from build123d import *

# Parameters (mm, degrees)
SKETCH1_R           = 23
SKETCH1_R_2         = 18
BOSS_EXTRUDE1_DEPTH = 11
SKETCH1_13_R        = 23
SKETCH1_13_R_2      = 18
SKETCH1_13_R_3      = 3
SKETCH1_13_R_4      = 5.25
BOSS_EXTRUDE2_DEPTH = 3
BOSS_EXTRUDE4_START = 3
SKETCH1_16_R        = 23
SKETCH1_16_R_2      = 18
SKETCH1_16_R_3      = 3
SKETCH1_16_R_4      = 5.25
SKETCH1_16_R_5      = 1.5
BOSS_EXTRUDE4_DEPTH = 3
SKETCH1_17_R        = 23
SKETCH1_17_R_2      = 18
BOSS_EXTRUDE5_DEPTH = 60
SKETCH2_R           = 1.5
CUT_EXTRUDE1_DEPTH  = 5
BOSS_EXTRUDE6_START = 6
SKETCH1_20_R        = 3
SKETCH1_20_R_2      = 1.5
BOSS_EXTRUDE6_DEPTH = 3
SKETCH1_21_R        = 23
SKETCH1_21_R_2      = 18
CUT_EXTRUDE4_DEPTH  = 23
SKETCH2_2_R         = 1.5
CUT_EXTRUDE5_DEPTH  = 9


with BuildPart() as part:
    # Sketch1 → Boss-Extrude1 (new body)
    with BuildSketch(Plane(origin=(0, 0, 0), x_dir=(0, 0, -1), z_dir=(1, 0, 0))):
        Circle(SKETCH1_R)
        Circle(SKETCH1_R_2, mode=Mode.SUBTRACT)
    extrude(amount=-BOSS_EXTRUDE1_DEPTH)

    # Sketch1_13 → Boss-Extrude2 (add)
    with BuildSketch(Plane(origin=(0, 0, 0), x_dir=(0, 0, -1), z_dir=(1, 0, 0))):
        Circle(SKETCH1_13_R)
        Circle(SKETCH1_13_R_2, mode=Mode.SUBTRACT)
        Circle(SKETCH1_13_R_2)
        with Locations((-8.5, 0)):
            Circle(SKETCH1_13_R_3, mode=Mode.SUBTRACT)
        with Locations((8.5, 0)):
            Circle(SKETCH1_13_R_3, mode=Mode.SUBTRACT)
        Circle(SKETCH1_13_R_4, mode=Mode.SUBTRACT)
        with Locations((0, -8.5)):
            Circle(SKETCH1_13_R_3, mode=Mode.SUBTRACT)
        with Locations((0, 8.5)):
            Circle(SKETCH1_13_R_3, mode=Mode.SUBTRACT)
    extrude(amount=BOSS_EXTRUDE2_DEPTH)

    # Sketch1_16 → Boss-Extrude4 (add)
    with BuildSketch(Plane(origin=(0, 0, 0), x_dir=(0, 0, -1), z_dir=(1, 0, 0)).offset(BOSS_EXTRUDE4_START)):
        Circle(SKETCH1_16_R)
        Circle(SKETCH1_16_R_2, mode=Mode.SUBTRACT)
        Circle(SKETCH1_16_R_2)
        with Locations((-8.5, 0)):
            Circle(SKETCH1_16_R_3, mode=Mode.SUBTRACT)
        with Locations((8.5, 0)):
            Circle(SKETCH1_16_R_3, mode=Mode.SUBTRACT)
        Circle(SKETCH1_16_R_4, mode=Mode.SUBTRACT)
        with Locations((0, -8.5)):
            Circle(SKETCH1_16_R_3, mode=Mode.SUBTRACT)
        with Locations((0, 8.5)):
            Circle(SKETCH1_16_R_3, mode=Mode.SUBTRACT)
        with Locations((0, 8.5)):
            Circle(SKETCH1_16_R_3)
        with Locations((0, 8.5)):
            Circle(SKETCH1_16_R_5, mode=Mode.SUBTRACT)
        with Locations((-8.5, 0)):
            Circle(SKETCH1_16_R_3)
        with Locations((-8.5, 0)):
            Circle(SKETCH1_16_R_5, mode=Mode.SUBTRACT)
        with Locations((0, -8.5)):
            Circle(SKETCH1_16_R_3)
        with Locations((0, -8.5)):
            Circle(SKETCH1_16_R_5, mode=Mode.SUBTRACT)
        with Locations((8.5, 0)):
            Circle(SKETCH1_16_R_3)
        with Locations((8.5, 0)):
            Circle(SKETCH1_16_R_5, mode=Mode.SUBTRACT)
    extrude(amount=BOSS_EXTRUDE4_DEPTH)

    # Sketch1_17 → Boss-Extrude5 (add)
    with BuildSketch(Plane(origin=(0, 0, 0), x_dir=(0, 0, -1), z_dir=(1, 0, 0))):
        Circle(SKETCH1_17_R)
        Circle(SKETCH1_17_R_2, mode=Mode.SUBTRACT)
    extrude(amount=BOSS_EXTRUDE5_DEPTH)

    # Sketch2 → Cut-Extrude1 (cut)
    with BuildSketch(Plane(origin=(60, 0, 0), x_dir=(0, 0, -1), z_dir=(1, 0, 0))):
        with Locations((0, 20.5)):
            Circle(SKETCH2_R)
        with Locations((20.5, 0)):
            Circle(SKETCH2_R)
        with Locations((0, -20.5)):
            Circle(SKETCH2_R)
        with Locations((-20.5, 0)):
            Circle(SKETCH2_R)
    extrude(amount=-CUT_EXTRUDE1_DEPTH, mode=Mode.SUBTRACT)

    # Sketch1_20 → Boss-Extrude6 (add)
    with BuildSketch(Plane(origin=(0, 0, 0), x_dir=(0, 0, -1), z_dir=(1, 0, 0)).offset(BOSS_EXTRUDE6_START)):
        with Locations((0, 8.5)):
            Circle(SKETCH1_20_R)
        with Locations((0, 8.5)):
            Circle(SKETCH1_20_R_2, mode=Mode.SUBTRACT)
        with Locations((-8.5, 0)):
            Circle(SKETCH1_20_R)
        with Locations((-8.5, 0)):
            Circle(SKETCH1_20_R_2, mode=Mode.SUBTRACT)
        with Locations((0, -8.5)):
            Circle(SKETCH1_20_R)
        with Locations((0, -8.5)):
            Circle(SKETCH1_20_R_2, mode=Mode.SUBTRACT)
        with Locations((8.5, 0)):
            Circle(SKETCH1_20_R)
        with Locations((8.5, 0)):
            Circle(SKETCH1_20_R_2, mode=Mode.SUBTRACT)
    extrude(amount=-BOSS_EXTRUDE6_DEPTH)

    # Sketch1_21 → Cut-Extrude4 (cut)
    with BuildSketch(Plane(origin=(0, 0, 0), x_dir=(0, 0, -1), z_dir=(1, 0, 0))):
        Circle(SKETCH1_21_R)
        Circle(SKETCH1_21_R_2, mode=Mode.SUBTRACT)
    extrude(amount=-CUT_EXTRUDE4_DEPTH, mode=Mode.SUBTRACT)

    # Sketch2_2 → Cut-Extrude5 (cut)
    with BuildSketch(Plane(origin=(60, 0, 0), x_dir=(0, 0, -1), z_dir=(1, 0, 0))):
        with Locations((0, 20.5)):
            Circle(SKETCH2_2_R)
        with Locations((20.5, 0)):
            Circle(SKETCH2_2_R)
        with Locations((0, -20.5)):
            Circle(SKETCH2_2_R)
        with Locations((-20.5, 0)):
            Circle(SKETCH2_2_R)
    extrude(amount=-CUT_EXTRUDE5_DEPTH, mode=Mode.SUBTRACT)


solid = part.part
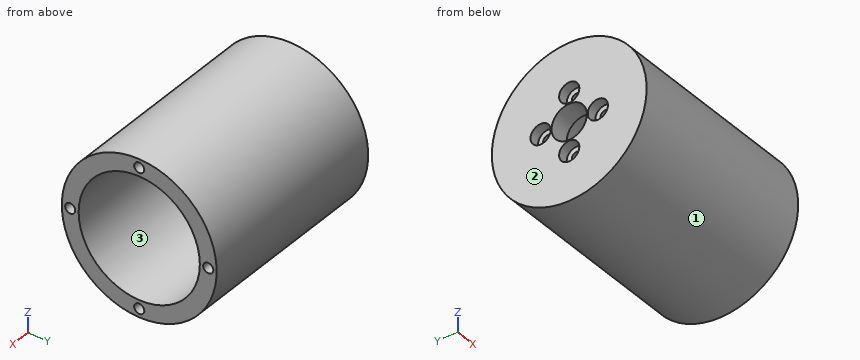
For this review, take the finished solid that the model builds, in its own axes (mm). Face numbers are marked on the shaded views. Round coordinates to 2 decimals unless told otherwise and drop trailing zeros. Loops run counter-clockwise (first coordinate to the right, second up) from the corner with the lowest first, then second, coordinate; pieces in that order, holes last. Notation, with made-up numbers: (-31, 79) - (22, 79) arc R26 ccw to (22, 111) - close; hole circle Ø1 at (-40, 60). An arc over 180 degrees is marked (long way). Use one line per item in the form item = value.
1) We need section C-C on x = 36. Write out the cut boundary in (y, z).
Solutions:
outline = circle Ø46 at (0, 0); hole circle Ø36 at (0, 0)
2) Mouldability with a two-part tool opening along Y and no side actions: class the marked faces 1, 2 and 3 as pulls with the +Y half, pulls with the -Y half, needs draft (parallel to the pull), parting line crosses it, or undercut.
Solutions:
face_1 = parting line crosses it
face_2 = needs draft
face_3 = undercut
3) We need section D-D on z = 0. State how many separate pieces and enclosed holes the cut face has, then the cut area to 3 significant figures.
Solutions:
separate_pieces = 4
enclosed_holes = 0
area = 645 mm2
4) We need section A-A on y = 8.5. Write out the cut boundary in (x, z), then the cut area to 3 significant figures.
Solutions:
outline = (0, -21.37) - (60, -21.37) - (60, -15.87) - (6, -15.87) - (6, -1.5) - (3, -1.5) - (3, -3) - (0, -3) - close; (0, 3) - (3, 3) - (3, 1.5) - (6, 1.5) - (6, 15.87) - (60, 15.87) - (60, 21.37) - (0, 21.37) - close
area = 824 mm2
5) Wall thickness on probe 1 along Y at (x, z) = (55, 0); probe 2 along Y at (x, z) = (4.6, 0); probe 3 along Y at (x, z) = (45, 0): over which ranges is each line inside the solid? List them lowest first.
Solutions:
probe_1 = -23 to -22, -19 to -18, 18 to 19, 22 to 23
probe_2 = -23 to -10, -7 to -5.25, 5.25 to 7, 10 to 23
probe_3 = -23 to -18, 18 to 23
6) Clearance check with flat-ended pins moving along their axes: P1, Ø3.5, axis at y = 0, z = 8.5, coming from the -X side; P2, Ø2.5, axis at y = 0, z = 8.5, coming from the -X side; P3, Ø2, axis at x = 50, z = 8.5, coming from the -Y side; P4, Ø1.5, axis at y = -0.5, z = -21, coming from the +X side. State where each tip first meets the part, or that it passes through.
Solutions:
P1 = 3
P2 = through
P3 = -21.74
P4 = 51
